Check sheet for the modelled part. Datum: model origin and axes. Units: mm. A direction names the side the tool comes from. Round coordinates to 2 decimals unless told otherwise and drop trailing zeros. Write each loop counter-clockwise with the first axis right and the second up, starting at its lowest first coordinate (ties: lowest second). Pieces come first, ordered by that corner, then holes. Notation, with made-up numbers: M 54,-4.75 L 81,-4.75 A17 ccw 81,4.25 Z; hole C -12,35.5 d2. An arc over 180 degrees is marked long. One line per item, written item: value.
from build123d import *

# Parameters (mm, degrees)
BOSS_EXTRUDE1_DEPTH        = 2.54
BOSS_EXTRUDE1_DEPTH_BACK   = 25.4
BOSS_EXTRUDE1_2_DEPTH      = 2.54
BOSS_EXTRUDE1_2_DEPTH_BACK = 25.4
CUT_EXTRUDE1_DEPTH         = 38.1
SKETCH5_R                  = 52.5
SKETCH5_R_2                = 40
CUT_EXTRUDE2_DEPTH         = 63.505162797
SKETCH6_W                  = 110.993636282
SKETCH6_H                  = 2.54
BOSS_EXTRUDE2_DEPTH        = 2
SKETCH7_W                  = 110.993636282
SKETCH7_H                  = 2.54
BOSS_EXTRUDE3_DEPTH        = 2
SKETCH8_W                  = 85.612929722
SKETCH8_H                  = 41.20835684
CUT_EXTRUDE4_DEPTH         = 2.54


with BuildPart() as part:
    # Sketch1 → Boss-Extrude1 (new, two sides: drawn at the far end of the back side and taken through both)
    with BuildSketch(Plane.XY.offset(-BOSS_EXTRUDE1_DEPTH_BACK)):
        with BuildLine():
            Line((-55.496818141, -9.53516), (-34.911270727, -9.53516))
            ThreePointArc((-34.911270727, -9.53516), (-36.19, 0), (-34.911270727, 9.53516))
            Line((-34.911270727, 9.53516), (-55.496818141, 9.53516))
            ThreePointArc((-55.496818141, 9.53516), (-56.31, 0), (-55.496818141, -9.53516))
        make_face()
    extrude(amount=BOSS_EXTRUDE1_DEPTH + BOSS_EXTRUDE1_DEPTH_BACK)


with BuildPart() as body_2:
    # Sketch1 → Boss-Extrude1 2 (new, two sides: drawn at the far end of the back side and taken through both)
    with BuildSketch(Plane.XY.offset(-BOSS_EXTRUDE1_2_DEPTH_BACK)):
        with BuildLine():
            Line((55.496818141, 9.53516), (34.911270727, 9.53516))
            ThreePointArc((34.911270727, 9.53516), (36.19, 0), (34.911270727, -9.53516))
            Line((34.911270727, -9.53516), (55.496818141, -9.53516))
            ThreePointArc((55.496818141, -9.53516), (56.31, 0), (55.496818141, 9.53516))
        make_face()
    extrude(amount=BOSS_EXTRUDE1_2_DEPTH + BOSS_EXTRUDE1_2_DEPTH_BACK)


with BuildPart() as cut_extrude1_tool:
    # Sketch3 → Cut-Extrude1 (new body)
    with BuildSketch(Plane.XY.offset(2.54)):
        with BuildLine():
            Line((39.730552161, 6.27), (31.319999693, 6.27))
            ThreePointArc((31.319999693, 6.27), (31.941435171, 0), (31.319999693, -6.27))
            Line((31.319999693, -6.27), (39.730552161, -6.27))
            ThreePointArc((39.730552161, -6.27), (40.22225348, 0), (39.730552161, 6.27))
        make_face()
        with BuildLine():
            Line((-31.319999693, 6.27), (-39.730552161, 6.27))
            ThreePointArc((-39.730552161, 6.27), (-40.22225348, 0), (-39.730552161, -6.27))
            Line((-39.730552161, -6.27), (-31.319999693, -6.27))
            ThreePointArc((-31.319999693, -6.27), (-31.941435171, 0), (-31.319999693, 6.27))
        make_face()
    extrude(amount=-CUT_EXTRUDE1_DEPTH)


with BuildPart() as part_1:
    add(part.part)

    # Cut-Extrude1: cut by cut_extrude1_tool
    add(cut_extrude1_tool.part, mode=Mode.SUBTRACT)


with BuildPart() as body_2_1:
    add(body_2.part)

    # Cut-Extrude1: cut by cut_extrude1_tool
    add(cut_extrude1_tool.part, mode=Mode.SUBTRACT)


with BuildPart() as cut_extrude2_tool:
    # Sketch5 → Cut-Extrude2 (new, through all)
    with BuildSketch(Plane.XY):
        Circle(SKETCH5_R)
        Circle(SKETCH5_R_2, mode=Mode.SUBTRACT)
    extrude(amount=-CUT_EXTRUDE2_DEPTH)


with BuildPart() as part_2:
    add(part_1.part)

    # Cut-Extrude2: cut by cut_extrude2_tool
    add(cut_extrude2_tool.part, mode=Mode.SUBTRACT)



with BuildPart() as body_2_2:
    add(body_2_1.part)

    # Cut-Extrude2: cut by cut_extrude2_tool
    add(cut_extrude2_tool.part, mode=Mode.SUBTRACT)


with BuildPart() as part_3:
    add(part_2.part)

    add(body_2_2.part)  # Boss-Extrude2 merges body 2
    # Sketch6 → Boss-Extrude2 (add)
    with BuildSketch(Plane.XZ.offset(9.53516)):
        with Locations((0, 1.27)):
            Rectangle(SKETCH6_W, SKETCH6_H)
    extrude(amount=BOSS_EXTRUDE2_DEPTH)

    # Sketch7 → Boss-Extrude3 (add)
    with BuildSketch(Plane(origin=(0, 9.53516, 0), x_dir=(1, 0, 0), z_dir=(0, 1, 0))):
        with Locations((0, -1.27)):
            Rectangle(SKETCH7_W, SKETCH7_H)
    extrude(amount=BOSS_EXTRUDE3_DEPTH)

    # Sketch8 → Cut-Extrude4 (cut)
    with BuildSketch(Plane(origin=(0, 0, -25.4), x_dir=(-1, 0, 0), z_dir=(0, 0, -1))):
        Rectangle(SKETCH8_W, SKETCH8_H)
    extrude(amount=-CUT_EXTRUDE4_DEPTH, mode=Mode.SUBTRACT)


solid = part_3.part
Q1. Sectioned sample at A-A on x = 21.5. Enter the section's corners in (y, z).
Completed:
outline: M -11.54,0 L -9.54,0 L -9.54,2.54 L -11.54,2.54 Z; M 9.54,0 L 11.54,0 L 11.54,2.54 L 9.54,2.54 Z
Q2. Depth check by flat-ended pin: P1, Ø2, axis at x = -35.5, z = -22, coming from the +Y side; P2, Ø6, axis at y = 7, z = -2, coming from the -X side; P3, Ø2, axis at y = -2.5, z = -11, coming from the -X side. Enter the tip coordinate at first touch or a pass-through.
Completed:
P1: y = 9.54
P2: x = -56.17
P3: x = -56.29
Q3. Sectioned sample at B-B on z = -13.25. Enter the section's corners in (x, y), and give its area (3 significant figures).
Completed:
outline: M -55.5,-9.54 L -51.63,-9.54 A52.5 cw -51.63,9.54 L -55.5,9.54 A56.31 ccw Z; M -39.51,-6.27 A40 ccw -38.85,-9.54 L -34.91,-9.54 A36.19 cw -35.64,-6.27 Z; M -39.51,6.27 L -35.64,6.27 A36.19 cw -34.91,9.54 L -38.85,9.54 A40 ccw Z; M 34.91,-9.54 L 38.85,-9.54 A40 ccw 39.51,-6.27 L 35.64,-6.27 A36.19 cw Z; M 34.91,9.54 A36.19 cw 35.64,6.27 L 39.51,6.27 A40 ccw 38.85,9.54 Z; M 51.63,-9.54 L 55.5,-9.54 A56.31 ccw 55.5,9.54 L 51.63,9.54 A52.5 cw Z
area: 197 mm^2
Q4. Draft check along X on faces 5 (the flat face through (-55.497, -11, 1)), 6 (the flat face through (55.497, 11, 1)), 7 (the cylindrical face through (35.32, -7.89, -10.34)). Enter one of: pulls with the +X half, pulls with the -X half, needs draft (parallel to the pull), parting line crosses it, or undercut.
Completed:
face 5: pulls with the -X half
face 6: pulls with the +X half
face 7: undercut
Q5. Access from +Z, -Z, +X, -X, +Y, -Y to the whole of each face (thin tool, end or side, straight path). Record for faces 1 (the flat face through (54, 9.535, -13)), 2 (the cylindrical face through (52.5, -0.1, -12.5)), 3 (the flat face through (37, 8, -22.86)), 4 (the cylindrical face through (-35.31, -7.93, -10.34)).
Completed:
face 1: -Z, +X, -X, +Y
face 2: -Z
face 3: -Z, +Y, -Y
face 4: +Z, -Z
Q6. Scan lines: line 1 (X direction, y = 8.5, z = -20.5); line 2 (X direction, y = -7, z = -3.25); line 3 (Z direction, x = 48, y = -9.5). Record each from-to range of solid material in increasing order. Write a range as [from, to].
Completed:
line 1: [-55.66, -51.81], [-39.09, -35.18], [35.18, 39.09], [51.81, 55.66]
line 2: [-55.87, -52.03], [-39.38, -35.51], [35.51, 39.38], [52.03, 55.87]
line 3: [0, 2.54]
Q7. Sectioned sample at D-D on y = 7.25. Enter the section's corners in (x, z), and give its area (3 significant figures).
Completed:
outline: M -55.84,-25.4 L -52,-25.4 L -52,0 L -39.34,0 L -39.34,-22.86 L -35.46,-22.86 L -35.46,2.54 L -55.84,2.54 Z; M 35.46,-22.86 L 39.34,-22.86 L 39.34,0 L 52,0 L 52,-25.4 L 55.84,-25.4 L 55.84,2.54 L 35.46,2.54 Z
area: 476 mm^2
Q8. Sectioned sample at C-C on y = -0.5. Enter the section's corners in (x, z).
Completed:
outline: M -56.31,-25.4 L -52.5,-25.4 L -52.5,0 L -40.22,0 L -40.22,2.54 L -56.31,2.54 Z; M 40.22,0 L 52.5,0 L 52.5,-25.4 L 56.31,-25.4 L 56.31,2.54 L 40.22,2.54 Z
